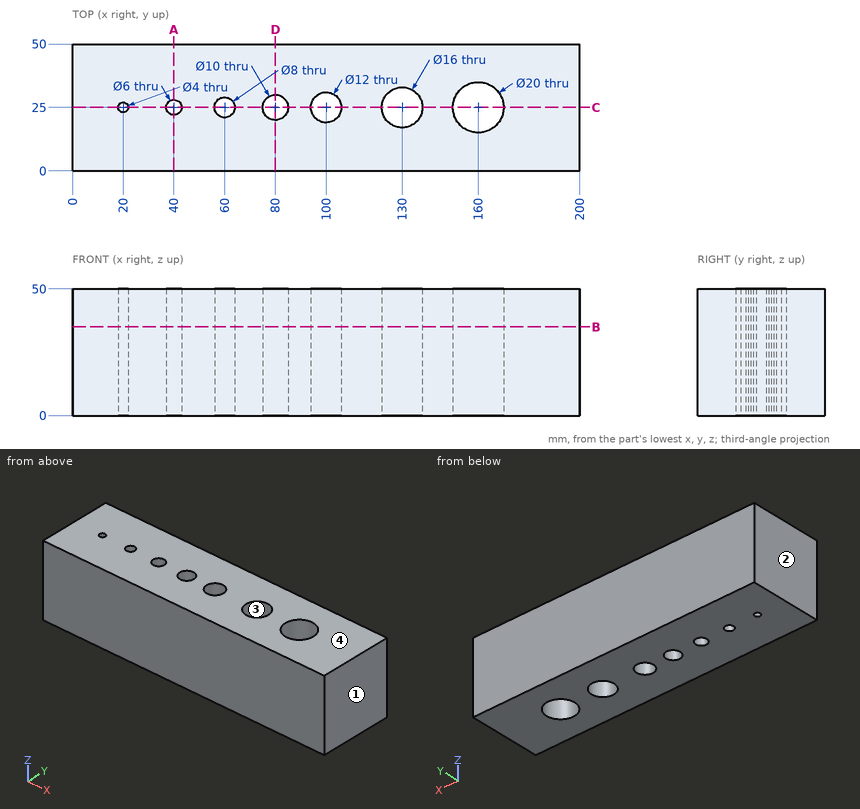
Drawing for the job (mm, zero at the part's lowest x, y, z). Round coordinates to 2 decimals unless told otherwise and drop trailing zeros. Write each loop counter-clockwise with the first axis right and the second up, starting at its lowest first coordinate (ties: lowest second). Pieces come first, ordered by that corner, then holes.
Item 1: Band-saw the part on B-B on z = 35. Write the cut outline in (x, y), then the cut area to 3 significant figures.
Filled in:
outline: (0, 0) - (200, 0) - (200, 50) - (0, 50) - close; hole circle Ø4 at (20, 25); hole circle Ø6 at (40, 25); hole circle Ø8 at (60, 25); hole circle Ø10 at (80, 25); hole circle Ø12 at (100, 25); hole circle Ø16 at (130, 25); hole circle Ø20 at (160, 25)
area: 9,200 mm2
Item 2: Mould opens along X. For the marked faces 1, 2, 3 and 4 say: released by +X, released by -X, zero draft, split by the parting line, or undercut.
Filled in:
face 1: released by +X
face 2: released by -X
face 3: undercut
face 4: zero draft
Item 3: Band-saw the part on D-D on x = 80. Write the cut outline in (y, z).
Filled in:
outline: (0, 0) - (20, 0) - (20, 50) - (0, 50) - close; (30, 0) - (50, 0) - (50, 50) - (30, 50) - close
Item 4: Band-saw the part on C-C on y = 25. Give the number of separate pieces and of enclosed holes in the cut face, then the cut area to 3 significant figures.
Filled in:
separate pieces: 8
enclosed holes: 0
area: 6,200 mm2
Item 5: Band-saw the part on A-A on x = 40. Write the cut outline in (y, z), then the cut area to 3 significant figures.
Filled in:
outline: (0, 0) - (22, 0) - (22, 50) - (0, 50) - close; (28, 0) - (50, 0) - (50, 50) - (28, 50) - close
area: 2,200 mm2
Item 6: Drill centre lines: L1, parallel to Y at x = 60, z = 30; L2, parallel to Y at x = 80, z = 27; L3, parallel to X at y = 31.5, z = 22. Where is each one in solid material? Low to high.
Filled in:
L1: y = 0 to 21, 29 to 50
L2: y = 0 to 20, 30 to 50
L3: x = 0 to 125.34, 134.66 to 152.4, 167.6 to 200
